Build history of the part. All positions in model axes, mm. Face numbers are marked on the shaded views. A direction names the side the tool comes from. Round coordinates to 2 decimals unless told otherwise and drop trailing zeros. Loops run counter-clockwise (first coordinate to the right, second up) from the corner with the lowest first, then second, coordinate; pieces in that order, holes last. Notation, with made-up numbers: M 42,84 L 73,84 A29 ccw 73,110 Z; hole C -14,58.25 d8. An arc over 180 degrees is marked long. Write each question's results on one line, items separated by ' | '. Start each with the question number.
```python
from build123d import *

# Parameters (mm, degrees)
F0_W     = 12
F0_H     = 12
F1_DEPTH = 4
F2_W     = 2
F2_H     = 12
F3_DEPTH = 8
F4_R     = 7.5
F5_DEPTH = 9


with BuildPart() as f1:
    # F0 (on Top) → F1 (new body)
    with BuildSketch(Plane.XY):
        Rectangle(F0_W, F0_H)
    extrude(amount=-F1_DEPTH)

    # F2 (on Top) → F3 (join)
    with BuildSketch(Plane.XY):
        with Locations((-5, 0)):
            Rectangle(F2_W, F2_H)
        with Locations((5, 0)):
            Rectangle(F2_W, F2_H)
    extrude(amount=-F3_DEPTH)

    # F4 (on Top) → F5 (join)
    with BuildSketch(Plane.XY):
        Circle(F4_R)
    extrude(amount=F5_DEPTH)


solid = f1.part
```
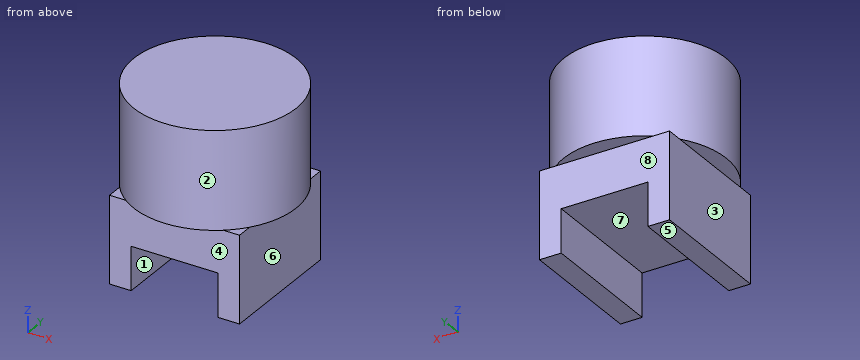
Item 1: Saw through at D-D, the plane z = -3.25. Give the cut face in (x, y).
Item 2: Saw through at C-C, the plane y = 0. Give the cut face in (x, z).
Item 3: Saw through at A-A, the plane z = -5. Give the cut face in (x, y), then the cut area to 3 significant figures.
Item 4: Drop flat-ended pins along their axis: pin 1 (1.7 mm diameter, centred on x = 2, y = -7, fed in from -Z); pin 2 (1.5 mm diameter, centred on x = -2.5, z = -4, fed in from +Y); pin 3 (2.5 mm diameter, centred on y = -2.5, z = -4.5, fed in from -X); pin 4 (9 mm diameter, centred on x = 0, z = -3.5, fed in from -Y). Give the stop position or say it passes through.
Item 5: Saw through at B-B, the plane x = 0. Give the cut face in (y, z), then the cut area to 3 significant figures.
Item 6: Mould opens along X. For the marked faces 6, 7 and 8 say: released by +X, released by -X, zero draft, split by the parting line, or undercut.
Item 7: Drill centre lines: line 1 along X through (y, z) = (-4, -5.25); line 2 along X through (y, z) = (-1.25, -2); line 3 along Z through (x, y) = (6.5, -2.75). Where is each one in solid material? Low to high. Write a range as [from, to].
Item 8: Tool access for the marked faces 1, 2, 3, 4 and 5: list every direction of +Z, -Z, +X, -X, +Y, -Y with a clear straight run to the whole face (end or side of a thin tool).
Working result:
1) outline: M -6,-6 L 6,-6 L 6,6 L -6,6 Z
2) outline: M -7.5,0 L -6,0 L -6,-8 L -4,-8 L -4,-4 L 4,-4 L 4,-8 L 6,-8 L 6,0 L 7.5,0 L 7.5,9 L -7.5,9 Z
3) outline: M -6,-6 L -4,-6 L -4,6 L -6,6 Z; M 4,-6 L 6,-6 L 6,6 L 4,6 Z | area: 48.0 mm²
4) pin 1: stops at z = 0 | pin 2: stops at y = 6 | pin 3: stops at x = -6 | pin 4: stops at y = -7.5
5) outline: M -7.5,0 L -6,0 L -6,-4 L 6,-4 L 6,0 L 7.5,0 L 7.5,9 L -7.5,9 Z | area: 183 mm²
6) face 6: released by +X | face 7: undercut | face 8: zero draft
7) line 1: x = [-6, -4], [4, 6] | line 2: x = [-6, 6] | line 3: z = [0, 9]
8) face 1: -Z, +Y, -Y | face 2: +Z | face 3: -Z, -X, +Y, -Y | face 4: -Z, +X, -X, -Y | face 5: -Z, +X, -X, +Y, -Y
